from build123d import *

# Parameters (mm, degrees)
EXTRUDE_1_DEPTH = 2.9


with BuildPart() as part:
    # 草图1 → 凸台-拉伸1 (new body)
    with BuildSketch(Plane.XY):
        Polygon((65, 0), (100, 0), (100, 130), (99, 130), (99, 132.9), (95, 132.9), (94, 132.9), (94, 130), (6, 130), (6, 132.9), (5, 132.9), (1, 132.9), (1, 130), (0, 130), (0, 0), (35, 0), (35, -3), (50, -3), (65, -3), align=None)
    extrude(amount=EXTRUDE_1_DEPTH)


solid = part.part
Verification items for the finished model (mm, model axes). A direction names the side the tool comes from. Give positions to 0.01 mm unless a question says otherwise; leave off trailing zeros. Loops run counter-clockwise (first coordinate to the right, second up) from the corner with the lowest first, then second, coordinate; pieces in that order, holes last. Notation, with made-up numbers: (4, 47.25) - (42, 47.25) arc R21 cw to (42, 53.25) - close; hole circle Ø9 at (67, 78.5). An arc over 180 degrees is marked (long way). Write item = value, one per line. Start each with the question number.
Q1. Cross-section at A-A, the plane z = 0.5. Enter the section's corners in (x, y), and give its area (3 significant figures).
Q2. Thickness scan on line 1 (Y direction, x = 38.5, z = 1.55); line 2 (Y direction, x = 69, z = 2.3). Record the ranges inside material, lowest first.
Q3. Tool access check on faces 1 (the face through (99, 131, 1)), 2 (the face through (17, 0, 1)), 3 (the face through (1, 131, 1)). Record the directions out of +Z, -Z, +X, -X, +Y, -Y that give a thin tool (end or side, any length) a straight path to the whole face; none if there is none.
Q4. Cross-section at B-B, the plane x = 81. Enter the section's corners in (y, z).
Q5. Mould release check, pull along X, two halves, no side actions. Record for faces 4 (the face through (0, 66, 1)), 5 (the face through (50, -3, 1)), 6 (the face through (94, 131, 1)): released by +X, released by -X, zero draft, split by the parting line, or undercut.
Q6. Depth check by flat-ended pin: P1, Ø0.9, axis at y = 132, z = 1.5, coming from the +X side; P2, Ø1, axis at x = 19.5, z = 2, coming from the -Y side; P3, Ø1.4, axis at x = 67, z = 1.5, coming from the +Y side. Enter the tip coordinate at first touch or a pass-through.
Answer key:
q1.outline = (0, 0) - (35, 0) - (35, -3) - (65, -3) - (65, 0) - (100, 0) - (100, 130) - (99, 130) - (99, 132.9) - (94, 132.9) - (94, 130) - (6, 130) - (6, 132.9) - (1, 132.9) - (1, 130) - (0, 130) - close
q1.area = 13,100 mm^2
q2.line_1 = -3 to 130
q2.line_2 = 0 to 130
q3.face_1 = +Z, -Z, +X, +Y
q3.face_2 = +Z, -Z, -X, -Y
q3.face_3 = +Z, -Z, -X, +Y
q4.outline = (0, 0) - (130, 0) - (130, 2.9) - (0, 2.9) - close
q5.face_4 = released by -X
q5.face_5 = zero draft
q5.face_6 = undercut
q6.P1 = 99
q6.P2 = 0
q6.P3 = 130
